Part model, mm, in its own coordinate system. Face numbers are marked on the shaded views. A direction names the side the tool comes from. Give positions to 0.01 mm unless a question says otherwise; leave off trailing zeros. Write each loop counter-clockwise with the first axis right and the second up, starting at its lowest first coordinate (ties: lowest second). Pieces come first, ordered by that corner, then holes.
from build123d import *

# Parameters (mm, degrees)
SKETCH1_R           = 5
BOSS_EXTRUDE1_DEPTH = 12


with BuildPart() as part:
    # Sketch1 → Boss-Extrude1 (new, symmetric)
    with BuildSketch(Plane.XY):
        with BuildLine():
            Line((-10, 41), (-10, 31))
            ThreePointArc((-10, 31), (0, 21), (10, 31))
            Line((10, 31), (10, 41))
            Line((10, 41), (47, 41))
            Line((47, 41), (57, 31))
            Line((57, 31), (57, 12))
            Line((57, 12), (43, 12))
            ThreePointArc((43, 12), (31, 0), (43, -12))
            Line((43, -12), (57, -12))
            Line((57, -12), (57, -31))
            Line((57, -31), (47, -41))
            Line((47, -41), (10, -41))
            Line((10, -41), (10, -31))
            ThreePointArc((10, -31), (0, -21), (-10, -31))
            Line((-10, -31), (-10, -41))
            Line((-10, -41), (-47, -41))
            Line((-47, -41), (-57, -31))
            Line((-57, -31), (-57, -12))
            Line((-57, -12), (-43, -12))
            ThreePointArc((-43, -12), (-31, 0), (-43, 12))
            Line((-43, 12), (-57, 12))
            Line((-57, 12), (-57, 31))
            Line((-57, 31), (-47, 41))
            Line((-47, 41), (-10, 41))
        make_face()
        with Locations((-47, 29)):
            Circle(SKETCH1_R, mode=Mode.SUBTRACT)
        with Locations(Location((47, 29, 0), (0, 0, 180))):
            Circle(SKETCH1_R, mode=Mode.SUBTRACT)
        with Locations(Location((-47, -29, 0), (0, 0, 180))):
            Circle(SKETCH1_R, mode=Mode.SUBTRACT)
        with Locations((47, -29)):
            Circle(SKETCH1_R, mode=Mode.SUBTRACT)
    extrude(amount=BOSS_EXTRUDE1_DEPTH, both=True)


solid = part.part
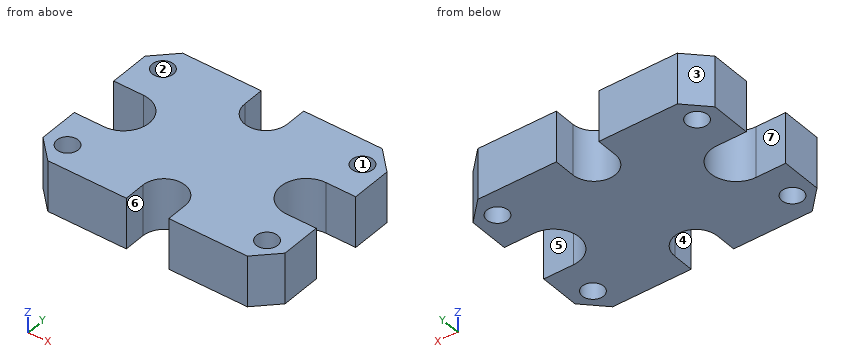
1) Saw through at D-D (y = -10). Write the cut outline in (x, z), and give its area (3 significant figures).
Check result:
outline: (-36.37, -12) - (36.37, -12) - (36.37, 12) - (-36.37, 12) - close
area: 1,750 mm2
2) Saw through at B-B (y = 27). Write the cut outline in (x, z).
Check result:
outline: (-57, -12) - (-51.58, -12) - (-51.58, 12) - (-57, 12) - close; (-42.42, -12) - (-9.17, -12) - (-9.17, 12) - (-42.42, 12) - close; (9.17, -12) - (42.42, -12) - (42.42, 12) - (9.17, 12) - close; (51.58, -12) - (57, -12) - (57, 12) - (51.58, 12) - close
3) Saw through at A-A (z = -4). Write the cut outline in (x, y), and give its area (3 significant figures).
Check result:
outline: (-57, -31) - (-47, -41) - (-10, -41) - (-10, -31) arc R10 cw to (10, -31) - (10, -41) - (47, -41) - (57, -31) - (57, -12) - (43, -12) arc R12 cw to (43, 12) - (57, 12) - (57, 31) - (47, 41) - (10, 41) - (10, 31) arc R10 cw to (-10, 31) - (-10, 41) - (-47, 41) - (-57, 31) - (-57, 12) - (-43, 12) arc R12 cw to (-43, -12) - (-57, -12) - close; hole circle Ø10 at (-47, -29); hole circle Ø10 at (-47, 29); hole circle Ø10 at (47, -29); hole circle Ø10 at (47, 29)
area: 7,000 mm2
4) Drill centre lines: L1, parallel to Y at x = -47, z = -0.5; L2, parallel to Y at x = 49, z = 6; L3, parallel to X at y = -25, z = -0.25. Where is each one in solid material? Low to high.
Check result:
L1: y = -41 to -34, -24 to -12, 12 to 24, 34 to 41
L2: y = -39 to -33.58, -24.42 to -12, 12 to 24.42, 33.58 to 39
L3: x = -57 to -50, -44 to -8, 8 to 44, 50 to 57
5) Flat gauge pins, fed straight in: P1, Ø11, axis at x = 53.5, z = 2.5, coming from the -Y side; P2, Ø6, axis at x = 43, y = 29, coming from the -Z side; P3, Ø11, axis at y = 37.5, z = -5.5, coming from the +X side; P4, Ø8, axis at y = 36, z = -2, coming from the -X side. Where does each tip first touch, or does it go through?
Check result:
P1: stops at y = -40
P2: stops at z = -12
P3: stops at x = 56
P4: stops at x = -56
6) 3-axis set-ups, long thin cutter, end or side, ignore diameter. For the marked faces 5, 6 and 7: which of +Z, -Z, +X, -X, +Y, -Y reach the whole face in a straight line?
Check result:
face 5: +Z, -Z, +X
face 6: +Z, -Z, -Y
face 7: +Z, -Z, -X
7) Saw through at C-C (y = 0). Write the cut outline in (x, z), and give its area (3 significant figures).
Check result:
outline: (-31, -12) - (31, -12) - (31, 12) - (-31, 12) - close
area: 1,490 mm2
8) Mould opens along Y. For the marked faces 1, 2, 3 and 4 say: +Y half, -Y half, draft (parallel to the pull), parting line (faces both ways), or undercut.
Check result:
face 1: undercut
face 2: undercut
face 3: +Y half
face 4: draft
